```python
from build123d import *

# Parameters (mm, degrees)
F1_DEPTH = 1320.8
F3_DEPTH = 812.801


with BuildPart() as f1:
    # F0 (on Top) → F1 (new body)
    with BuildSketch(Plane.XY):
        Polygon((812.8, 0), (0, 0), (0, -330.2), (177.8, -660.4), (635, -660.4), (812.8, -330.2), align=None)
    extrude(amount=F1_DEPTH)

    # F2 (on face) → F3 (cut, through all)
    with BuildSketch(Plane.YZ.offset(812.8)):
        Polygon((0, 1320.8), (-660.393178, 1323.801782), (0, 812.8), align=None)
    extrude(amount=-F3_DEPTH, mode=Mode.SUBTRACT)


solid = f1.part
```
Geometry check sheet. Reference: the model listing, model coordinates, mm. Round coordinates to 2 decimals unless told otherwise and drop trailing zeros. Order: outer loops, then holes, each group sorted by start corner. A loop starts at its lowest first (then second) coordinate and runs counter-clockwise, first axis right, second up. Notation, with made-up numbers: (13.5, 18.5) - (70.5, 18.5) arc R19 cw to (70.5, 42.5) - close; hole circle Ø11 at (0, 59.5). An arc over 180 degrees is marked (long way). Use a Markdown table: item, result. Add a question column.
1) Section check D-D (z = 1161). Record the cut outline in (x, y), then the cut area to 3 significant figures.
2) Gauge pin test, flat ends, axial feed: P1, Ø1.5, axis at x = 449, z = 244.5, coming from the +Y side; P2, Ø6, axis at x = 717, z = 1001.5, coming from the -Y side. Record the tip position at first contact, or that the pin passes through.
3) Section check C-C (y = -509). Record the cut outline in (x, z), then the cut area to 3 significant figures.
4) Mould release check, pull along X, two halves, no side actions. Record for faces 1 (the flat face through (812.8, -167, 527)), 2 (the flat face through (0, -163, 408)), 3 (the flat face through (412, 0, 401)): released by +X, released by -X, zero draft, split by the parting line, or undercut.
5) Section check B-B (z = 441.5). Record the cut outline in (x, y), then the cut area to 3 significant figures.
6) Section check A-A (x = 309). Record the cut outline in (y, z).
7) Thickness scan on line 1 along Z through (x, y) = (620, -510.5); line 2 along Z through (x, y) = (331.5, -45.5); line 3 along Y through (x, z) = (392.5, 893). Record the ranges inside material, lowest first.
Established:
| question | item | result |
|---|---|---|
| 1 | outline | (64.51, -450) - (177.8, -660.4) - (635, -660.4) - (748.29, -450) - close |
| 1 | area | 120,000 mm2 |
| 2 | P1 | y = 0 |
| 2 | P2 | y = -513.69 |
| 3 | outline | (96.28, 0) - (716.52, 0) - (716.52, 1206.66) - (96.28, 1206.66) - close |
| 3 | area | 748,000 mm2 |
| 4 | face 1 | released by +X |
| 4 | face 2 | released by -X |
| 4 | face 3 | zero draft |
| 5 | outline | (0, -330.2) - (177.8, -660.4) - (635, -660.4) - (812.8, -330.2) - (812.8, 0) - (0, 0) - close |
| 5 | area | 478,000 mm2 |
| 6 | outline | (-660.4, 0) - (0, 0) - (0, 812.8) - (-656.51, 1320.8) - (-660.4, 1320.8) - close |
| 7 | line 1 | 0 to 1207.82 |
| 7 | line 2 | 0 to 848.01 |
| 7 | line 3 | -660.4 to -103.65 |
